```python
from build123d import *

# Parameters (mm, degrees)
SKETCH_2_R          = 1.5
CUT_EXTRUDE_1_DEPTH = 30


with BuildPart() as part:
    # 草图1 → 旋转1 (revolve)
    with BuildSketch(Plane.XY, mode=Mode.PRIVATE) as revolve_1_sk:
        Polygon((-3.575, 15), (3.575, 15), (3.575, 8.2), (6.575, 8.2), (6.575, 23), (3.575, 23), (3.575, 17), (-3.575, 17), (-3.575, 23), (-6.575, 23), (-6.575, 8.2), (-3.575, 8.2), align=None)
    revolve(revolve_1_sk.sketch.rotate(Axis((0, 0, 0), (1, 0, 0)), 90), axis=Axis((0, 0, 0), (1, 0, 0)))

    # 草图2 → 切除-拉伸1 (cut)
    with BuildSketch(Plane.ZY.offset(6.575)):
        with Locations((20, 0)):
            Circle(SKETCH_2_R)
        with Locations((-20, 0)):
            Circle(SKETCH_2_R)
    extrude(amount=-CUT_EXTRUDE_1_DEPTH, mode=Mode.SUBTRACT)


solid = part.part
```
Here's how the part is built. I have some questions about the finished solid (model axes, mm). A direction names the side the tool comes from. Round coordinates to 2 decimals unless told otherwise and drop trailing zeros. Order: outer loops, then holes, each group sorted by start corner. A loop starts at its lowest first (then second) coordinate and runs counter-clockwise, first axis right, second up. Notation, with made-up numbers: (-1.5, 10.25) -> (6.5, 10.25) arc R36 cw to (6.5, 49.25) -> close; hole circle Ø8 at (65.25, 9). An arc over 180 degrees is marked (long way). Use a Markdown table: item, result. Add a question column.
(1) I need wall thicknesses on line 1 along X through (y, z) = (18, -2) (3 decimals); line 2 along Z through (x, y) = (-5.25, 0.5); line 3 along Y through (x, z) = (-4.6, 0). Which ranges of each line are inside material? Lowest first, please.
(2) Suppose I cut it at D-D, the plane x = -1.5. Please give me the cut outline in (y, z), and give its area (3 significant figures).
(3) If we mould it in two halves opening along X, with no side actions, what happens to faces 3 (the face through (-6.575, 0, 10)), 4 (the face through (-5.1, 0.07, -21.5)), 5 (the face through (-3.575, 6, -6)), 6 (the face through (6.575, 0, -10))? For each: released by +X, released by -X, zero draft, split by the parting line, or undercut.
(4) Suppose I cut it at B-B, the plane z = 0. Please give me the cut outline in (x, y) (3 decimals), and give its area (3 significant figures).
(5) For pin 1 Ø15 at (y, z) = (0, 0) entering from -X; pin 2 Ø2 at (x, z) = (3.5, -0.5) entering from -Y; pin 3 Ø3 at (x, y) = (-4.5, 4) entering from +Z; pin 4 Ø3 at (x, z) = (1, -9) entering from +Y, each with a flat end and sliding along its axis, tell me the tip position at first contact or that it passes through.
(6) Suppose I cut it at C-C, the plane z = -20. Please give me the cut outline in (x, y) (3 decimals), and give its area (3 significant figures).
(7) For faces 1 (the face through (3.575, 6, 6)), 2 (the face through (-5.1, 0.07, 18.5)), which set-ups out of +Z, -Z, +X, -X, +Y, -Y let a thin tool reach every point of the face, with its end or its side?
(8) Suppose I cut it at A-A, the plane y = -19.5. Please give me the cut outline in (x, z) (3 decimals), and give its area (3 significant figures).
Verdict:
| question | item | result |
|---|---|---|
| 1 | line 1 | -6.575 to -3.575, 3.575 to 6.575 |
| 1 | line 2 | -22.99 to -21.41, -18.59 to -8.18, 8.18 to 18.59, 21.41 to 22.99 |
| 1 | line 3 | -23 to -8.2, 8.2 to 23 |
| 2 | outline | circle Ø34 at (0, 0); hole circle Ø30 at (0, 0) |
| 2 | area | 201 mm2 |
| 3 | face 3 | released by -X |
| 3 | face 4 | zero draft |
| 3 | face 5 | undercut |
| 3 | face 6 | released by +X |
| 4 | outline | (-6.575, -23) -> (-3.575, -23) -> (-3.575, -17) -> (3.575, -17) -> (3.575, -23) -> (6.575, -23) -> (6.575, -8.2) -> (3.575, -8.2) -> (3.575, -15) -> (-3.575, -15) -> (-3.575, -8.2) -> (-6.575, -8.2) -> close; (-6.575, 8.2) -> (-3.575, 8.2) -> (-3.575, 15) -> (3.575, 15) -> (3.575, 8.2) -> (6.575, 8.2) -> (6.575, 23) -> (3.575, 23) -> (3.575, 17) -> (-3.575, 17) -> (-3.575, 23) -> (-6.575, 23) -> close |
| 4 | area | 206 mm2 |
| 5 | pin 1 | through |
| 5 | pin 2 | y = -23 |
| 5 | pin 3 | z = 22.86 |
| 5 | pin 4 | y = 15.26 |
| 6 | outline | (-6.575, -11.358) -> (-3.575, -11.358) -> (-3.575, -1.5) -> (-6.575, -1.5) -> close; (-6.575, 1.5) -> (-3.575, 1.5) -> (-3.575, 11.358) -> (-6.575, 11.358) -> close; (3.575, -11.358) -> (6.575, -11.358) -> (6.575, -1.5) -> (3.575, -1.5) -> close; (3.575, 1.5) -> (6.575, 1.5) -> (6.575, 11.358) -> (3.575, 11.358) -> close |
| 6 | area | 118 mm2 |
| 7 | face 1 | none |
| 7 | face 2 | +X, -X |
| 8 | outline | (-6.575, -12.196) -> (-3.575, -12.196) -> (-3.575, 12.196) -> (-6.575, 12.196) -> close; (3.575, -12.196) -> (6.575, -12.196) -> (6.575, 12.196) -> (3.575, 12.196) -> close |
| 8 | area | 146 mm2 |
